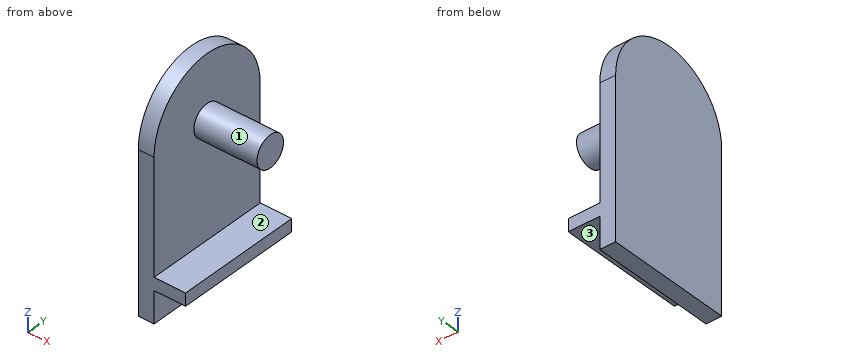
from build123d import *

# Parameters (mm, degrees)
BOSS_EXTRUDE1_DEPTH = 5
SKETCH2_W           = 40
SKETCH2_H           = 4
BOSS_EXTRUDE2_DEPTH = 10
SKETCH3_R           = 5
BOSS_EXTRUDE3_DEPTH = 20


with BuildPart() as part:
    # Sketch1 → Boss-Extrude1 (new body)
    with BuildSketch(Plane.YZ):
        with BuildLine():
            Line((20, 0), (20, -50))
            Line((20, -50), (-20, -50))
            Line((-20, -50), (-20, 0))
            ThreePointArc((-20, 0), (0, 20), (20, 0))
        make_face()
    extrude(amount=BOSS_EXTRUDE1_DEPTH)

    # Sketch2 → Boss-Extrude2 (add)
    with BuildSketch(Plane.YZ.offset(5)):
        with Locations((0, -38)):
            Rectangle(SKETCH2_W, SKETCH2_H)
    extrude(amount=BOSS_EXTRUDE2_DEPTH)

    # Sketch3 → Boss-Extrude3 (add)
    with BuildSketch(Plane.YZ.offset(5)):
        with Locations(Location((0, 0, 0), (0, 0, 270))):
            Circle(SKETCH3_R)
    extrude(amount=BOSS_EXTRUDE3_DEPTH)


solid = part.part
Design review of the part built by this model. Coordinates are the model's own, in mm. Face numbers are marked on the shaded views. A direction names the side the tool comes from. Give positions to 0.01 mm unless a question says otherwise; leave off trailing zeros. Loops run counter-clockwise (first coordinate to the right, second up) from the corner with the lowest first, then second, coordinate; pieces in that order, holes last. Notation, with made-up numbers: (19, -9.5) - (56, -9.5) arc R31 ccw to (56, 15.5) - close; hole circle Ø4 at (16.25, 32). An arc over 180 degrees is marked (long way). Write item = value, one per line.
1) Take a section at B-B on y = 0. State the section outline as (x, z) points, and give its area (3 significant figures).
Result sheet:
outline = (0, -50) - (5, -50) - (5, -40) - (15, -40) - (15, -36) - (5, -36) - (5, -5) - (25, -5) - (25, 5) - (5, 5) - (5, 20) - (0, 20) - close
area = 590 mm2
2) Tool access review of the marked faces 1, 2 and 3: name each direction out of +Z, -Z, +X, -X, +Y, -Y from which nothing blocks a thin tool from reaching the whole face with its end or side.
Result sheet:
face_1 = +X
face_2 = +X, +Y, -Y
face_3 = -Z, +X, +Y, -Y
3) To check wall thickness, follow line 1 (X direction, y = 11.5, z = -7.5); line 2 (Z direction, x = 6.75, y = 6.5); line 3 (Z direction, x = 13.75, y = 3.5). State the ranges of each line that lie inside material, in increasing order.
Result sheet:
line_1 = 0 to 5
line_2 = -40 to -36
line_3 = -40 to -36, -3.57 to 3.57
4) Clearance check with flat-ended pins moving along their axes: pin 1 Ø2 at (y, z) = (9, -38) entering from +X; pin 2 Ø5 at (y, z) = (6, 12.5) entering from +X; pin 3 Ø4 at (x, z) = (18, -42) entering from -Y; pin 4 Ø1 at (x, y) = (8, 8.5) entering from -Z. State where each tip first meets the part, or that it passes through.
Result sheet:
pin_1 = 15
pin_2 = 5
pin_3 = through
pin_4 = -40
5) Take a section at C-C on z = -8. State the section outline as (x, y) points.
Result sheet:
outline = (0, -20) - (5, -20) - (5, 20) - (0, 20) - close
6) Take a section at A-A on x = 13. State the section outline as (y, z) points, and give its area (3 significant figures).
Result sheet:
outline = (-20, -40) - (20, -40) - (20, -36) - (-20, -36) - close; circle Ø10 at (0, 0)
area = 239 mm2
7) Take a section at D-D on x = 23.25. State the section outline as (y, z) points, and give its area (3 significant figures).
Result sheet:
outline = circle Ø10 at (0, 0)
area = 78.5 mm2
